Part print with two shaded views. Sizes in mm from the minimum x, y, z corner. Coordinates: 2 decimals unless noted, no trailing zeros. Loops run counter-clockwise (first coordinate to the right, second up) from the corner with the lowest first, then second, coordinate; pieces in that order, holes last.
Item 1: Cut at A-A (x = 1.4). List the corners of the cut face in (y, z), and give its area (3 significant figures).
Item 2: Cut at B-B (z = 21.25). List the corners of the cut face in (x, y).
Item 3: Flat gauge pins, fed straight in: pin 1 (8 mm diameter, centred on y = 167, z = 19.5, fed in from -X); pin 2 (1.5 mm diameter, centred on x = 0.5, z = 9, fed in from -Y). Where does each tip first touch, or does it go through?
Item 4: Drill centre lines: line 1 along Y through (x, z) = (1.8, 12.5); line 2 along Z through (x, y) = (2.35, 252.5); line 3 along Z through (x, y) = (0.3, 252). Where is each one in solid material? Low to high.
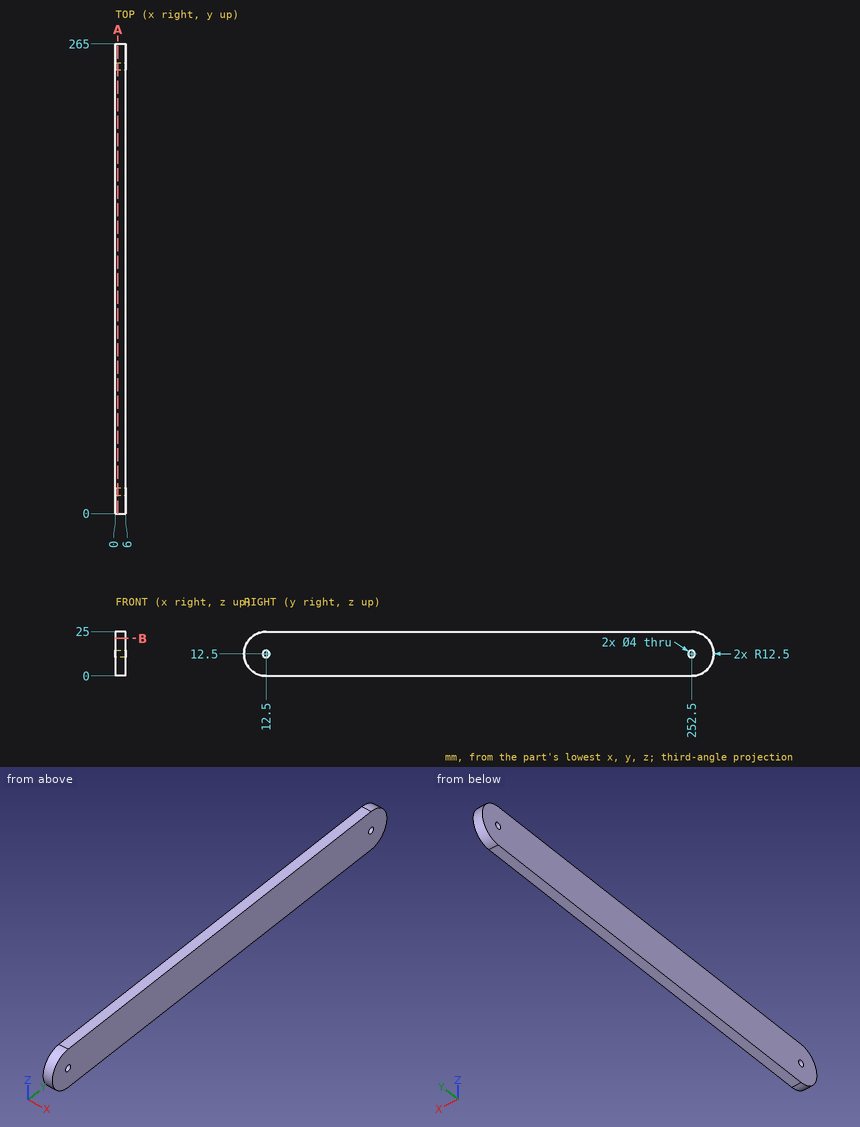
Filled sheet:
1. outline: (12.5, 0) - (252.5, 0) arc R12.5 ccw to (252.5, 25) - (12.5, 25) arc R12.5 ccw to start; hole circle Ø4 at (12.5, 12.5); hole circle Ø4 at (252.5, 12.5)
1. area: 6,470 mm2
2. outline: (0, 3.57) - (6, 3.57) - (6, 261.43) - (0, 261.43) - close
3. pin 1: stops at x = 0
3. pin 2: stops at y = 0.31
4. line 1: y = 0 to 10.5, 14.5 to 250.5, 254.5 to 265
4. line 2: z = 0 to 10.5, 14.5 to 25
4. line 3: z = 0 to 10.56, 14.44 to 25
